from build123d import *

# Parameters (mm, degrees)
BOSS_EXTRUDE1_DEPTH = 25
SKETCH2_R           = 1.25
BOSS_EXTRUDE2_DEPTH = 5
SKETCH3_R           = 2.5
CUT_EXTRUDE1_DEPTH  = 56.436901068
CHAMFER1_SIZE       = 2
CUT_EXTRUDE2_DEPTH  = 2
CHAMFER2_SIZE       = 3
SKETCH5_W           = 0.5
SKETCH5_H           = 47
CUT_EXTRUDE3_DEPTH  = 56.093103017
CHAMFER3_SIZE       = 10


with BuildPart() as part:
    # Sketch1 → Boss-Extrude1 (new body)
    with BuildSketch(Plane.XY):
        Polygon((-11.25, 0), (11.25, 0), (11.25, -10), (13, -10), (22, 0), (22, 6), (-22, 6), (-22, 0), (-13, -10), (-11.25, -10), align=None)
    extrude(amount=BOSS_EXTRUDE1_DEPTH)

    # Sketch2 → Boss-Extrude2 (add)
    with BuildSketch(Plane(origin=(22, 0, 0), x_dir=(0, 0, -1), z_dir=(1, 0, 0))):
        Polygon((-25, 6), (0, 6), (0, 8.5), (47, 8.5), (47, 25.5), (-25, 25.5), align=None)
        with Locations((-19, 17)):
            Circle(SKETCH2_R, mode=Mode.SUBTRACT)
        with Locations((41, 17)):
            Circle(SKETCH2_R, mode=Mode.SUBTRACT)
    extrude(amount=-BOSS_EXTRUDE2_DEPTH)

    # Sketch3 → Cut-Extrude1 (cut, through all)
    with BuildSketch(Plane(origin=(0, 6, 0), x_dir=(1, 0, 0), z_dir=(0, 1, 0))):
        with Locations(Location((0, -12.5, 0), (0, 0, 270))):
            Circle(SKETCH3_R)
    extrude(amount=-CUT_EXTRUDE1_DEPTH, mode=Mode.SUBTRACT)

    # Chamfer1
    chamfer1_edges = [part.edges().sort_by_distance(p)[0] for p in [
        (0, 6, 10),
    ]]
    chamfer(chamfer1_edges, length=CHAMFER1_SIZE)

    # Sketch4 → Cut-Extrude2 (cut)
    with BuildSketch(Plane(origin=(22, 0, 0), x_dir=(0, 0, -1), z_dir=(1, 0, 0))):
        Polygon((-16, 18.732050808), (-16, 15.267949192), (-19, 13.535898385), (-22, 15.267949192), (-22, 18.732050808), (-19, 20.464101615), align=None)
    cut_extrude2 = extrude(amount=-CUT_EXTRUDE2_DEPTH, mode=Mode.SUBTRACT)

    # Mirror1: Cut-Extrude2 across plane
    add(cut_extrude2.mirror(Plane.XY.offset(-11)), mode=Mode.SUBTRACT)

    # Chamfer2
    chamfer2_edges = [part.edges().sort_by_distance(p)[0] for p in [
        (17, 6, 12.5),
    ]]
    chamfer(chamfer2_edges, length=CHAMFER2_SIZE)

    # Sketch5 → Cut-Extrude3 (cut, through all)
    with BuildSketch(Plane.XZ.offset(-8.5)):
        with Locations((16.75, -23.5)):
            Rectangle(SKETCH5_W, SKETCH5_H)
    extrude(amount=-CUT_EXTRUDE3_DEPTH, mode=Mode.SUBTRACT)

    # Chamfer3
    chamfer3_edges = [part.edges().sort_by_distance(p)[0] for p in [
        (19.5, 8.5, 0),
    ]]
    chamfer(chamfer3_edges, length=CHAMFER3_SIZE)


solid = part.part
Could you check a few things on this model? Use its own coordinates, in mm. A direction names the side the tool comes from. Give positions to 0.01 mm unless a question says otherwise; leave off trailing zeros. Order: outer loops, then holes, each group sorted by start corner. A loop starts at its lowest first (then second) coordinate and runs counter-clockwise, first axis right, second up.
1. For faces 1 (the flat face through (20, 17, -47)), 2 (the flat face through (21, 14.4, -42.5)), 3 (the flat face through (11.25, -5, 12)), which set-ups out of +Z, -Z, +X, -X, +Y, -Y let a thin tool reach every point of the face, with its end or its side?
2. Suppose I cut it at A-A (y = 17). List the corners of the cut face in (x, z) for me.
3. We'd pull the mould along Z, two halves only. Please class faces 4 (the flat face through (21, 14.4, 20.5)), 5 (the flat face through (19.5, 3.4, -4.9)), 6 (the flat face through (12, -10, 12)): pulls with the +Z half, pulls with the -Z half, needs draft (parallel to the pull), parting line crosses it, or undercut.
4. Will these pins go through, and if not, where does the flat tip stop? P1, Ø3, axis at y = -6, z = 15, coming from the +X side; P2, Ø12, axis at y = -1, z = -18.5, coming from the +X side; P3, Ø18, axis at x = 2, z = 11.5, coming from the -Y side; P4, Ø5, axis at x = 16, y = 17, coming from the +Z side.
5. I need wall thicknesses on L1, parallel to Y at x = 19, z = -41; L2, parallel to X at y = 1.7, z = 12.5; L3, parallel to X at y = 23.5, z = -7.5. Which ranges of each line are inside material? Lowest first, please.
6. Suppose I cut it at B-B (x = 0). List the corners of the cut face in (y, z) for me.
7. Suppose I cut it at C-C (z = 12.5). List the corners of the cut face in (x, y) for me, plus the area to 3 significant figures.
8. Suppose I cut it at D-D (x = 18). List the corners of the cut face in (y, z) for me.
Solved:
1. face 1: -Z, +X, -X, +Y, -Y
1. face 2: +X
1. face 3: +Z, -Z, -Y
2. outline: (17, -47) - (22, -47) - (22, -44) - (20, -44) - (20, -42.25) - (17, -42.25) - close; (17, -39.75) - (20, -39.75) - (20, -38) - (22, -38) - (22, 16) - (20, 16) - (20, 17.75) - (17, 17.75) - close; (17, 20.25) - (20, 20.25) - (20, 22) - (22, 22) - (22, 25) - (17, 25) - close
3. face 4: undercut
3. face 5: pulls with the -Z half
3. face 6: needs draft
4. P1: stops at x = 17.95
4. P2: passes through
4. P3: stops at y = 0
4. P4: stops at z = 25
5. L1: y = 8.5 to 15.75, 18.25 to 25.5
5. L2: x = -22 to -2.5, 2.5 to 22
5. L3: x = 17 to 22
6. outline: (0, 0) - (6, 0) - (6, 8) - (4, 10) - (0, 10) - close; (0, 15) - (4, 15) - (6, 17) - (6, 25) - (0, 25) - close
7. outline: (-22, 0) - (-13, -10) - (-11.25, -10) - (-11.25, 0) - (-2.5, 0) - (-2.5, 4) - (-4.5, 6) - (-22, 6) - close; (2.5, 0) - (11.25, 0) - (11.25, -10) - (13, -10) - (22, 0) - (22, 25.5) - (17, 25.5) - (17, 9) - (14, 6) - (4.5, 6) - (2.5, 4) - close
7. area: 457 mm2
8. outline: (-4.44, 0) - (-1.5, 0) - (8.5, -10) - (8.5, -47) - (25.5, -47) - (25.5, 25) - (-4.44, 25) - close; hole circle Ø2.5 at (17, -41); hole circle Ø2.5 at (17, 19)
